Check sheet for the modelled part. Datum: model origin and axes. Units: mm. Face numbers are marked on the shaded views. A direction names the side the tool comes from. Coordinates: 2 decimals unless noted, no trailing zeros. Write each loop counter-clockwise with the first axis right and the second up, starting at its lowest first coordinate (ties: lowest second). Pieces come first, ordered by that corner, then holes. Notation, with made-up numbers: M -18,6.25 L 15,6.25 A19 cw 15,36.25 Z; hole C 31,55.25 d2. An arc over 180 degrees is marked long. Answer as CSV lines item,"result".
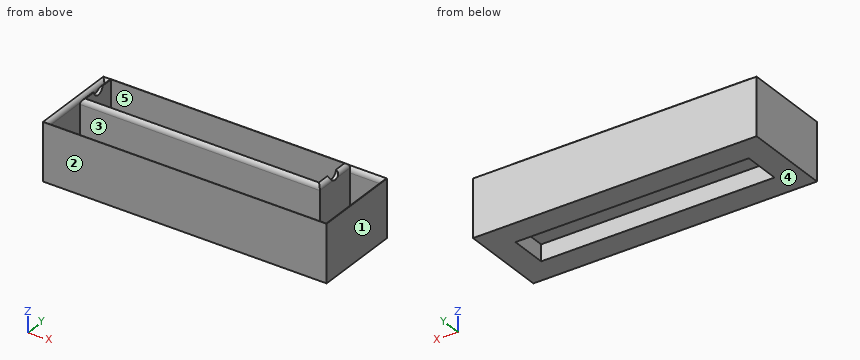
from build123d import *

# Parameters (mm, degrees)
F0_W          = 260
F0_H          = 80
F1_DEPTH      = 1
F2_W          = 10
F2_H          = 10
F3_DEPTH      = 50
F4_T          = 1
F4_T3_DEPTH   = 12
F4_T5_DEPTH   = 12
F4_T7_DEPTH   = 12
F4_T9_DEPTH   = 12
F5_W          = 260
F5_H          = 80
F6_DEPTH      = 3
F7_W          = 260
F7_H          = 80
F7_W_2        = 254
F7_H_2        = 74
F8_DEPTH      = 50
F9_W          = 220
F9_H          = 40
F10_DEPTH     = 67
F11_W         = 214
F11_H         = 34
F12_DEPTH     = 52
F13_W         = 214
F13_H         = 34
F14_DEPTH     = 15
F15_T1_DEPTH  = 245
F15_T3_DEPTH  = 65
F15_T5_DEPTH  = 254
F15_T7_DEPTH  = 74
F15_T13_DEPTH = 86.5
F15_T19_DEPTH = 266.5
F15_T28_DEPTH = 86.5
F15_T34_DEPTH = 266.5
F15_T43_DEPTH = 266.5
F15_T49_DEPTH = 86.5
F15_T58_DEPTH = 86.5
F15_T64_DEPTH = 266.5
F16_R         = 5.7285158572
F17_DEPTH     = 500
F18_W         = 260
F18_H         = 80
F19_DEPTH     = 51


# Not quite as in the source:
# - a fillet or chamfer that OpenCascade refuses, or shapes differently, is made with other operations: its cross-section is extruded or revolved along the edge and cut away or added
# - a shell that OpenCascade refuses in one call is made with other operations: the cavity is built on its own and cut out


with BuildPart() as f1:
    # F0 (on Top) → F1 (new body)
    with BuildSketch(Plane.XY):
        Rectangle(F0_W, F0_H)
    extrude(amount=F1_DEPTH)

    # F2 (on face) → F3 (join)
    with BuildSketch(Plane.XY.offset(1)):
        with Locations((-125, 35)):
            Rectangle(F2_W, F2_H)
        with Locations((125, 35)):
            Rectangle(F2_W, F2_H)
        with Locations((-125, -35)):
            Rectangle(F2_W, F2_H)
        with Locations((125, -35)):
            Rectangle(F2_W, F2_H)
    extrude(amount=F3_DEPTH)

    # F4: shell of thickness 1, made by hand


with BuildPart() as f4_core1:
    # F4_t2: copy of F1
    add(f1.part)

    # the walls: a layer under each face that stays
    f4_faces = [f4_core1.faces().sort_by_distance(p)[0] for p in [
        (121.3333333333, 40, 49.3),
        (-121.3333333333, -40, 49.3),
        (125, -35, 51),
        (125, -30, 26),
        (120, -35, 26),
        (-120, -35, 26),
        (-125, -30, 26),
        (-125, -35, 51),
        (-130, 34.2857142857, 47.3571428571),
        (-125, 30, 26),
        (-125, 35, 51),
        (-120, 35, 26),
        (0, 0, 1),
        (125, 30, 26),
        (120, 35, 26),
        (125, 35, 51),
        (130, -34.2857142857, 47.3571428571),
    ]]
    thicken(f4_faces, amount=-F4_T, mode=Mode.SUBTRACT)

    # F4_s4 → F4_t3 (cut)
    with BuildSketch(Plane.YZ.offset(119)):
        Polygon((-29.99, 1.01), (-31, 1), (-31, 0), (-30, 0), align=None)
        Polygon((29.99, 1.01), (30, 0), (31, 0), (31, 1), align=None)
    extrude(amount=F4_T3_DEPTH, mode=Mode.SUBTRACT)

    # F4_s6 → F4_t5 (cut)
    with BuildSketch(Plane.XZ.offset(29)):
        Polygon((119.99, 1.01), (121, 1), (121, 0), (120, 0), align=None)
        Polygon((-119.99, 1.01), (-121, 1), (-121, 0), (-120, 0), align=None)
    extrude(amount=F4_T5_DEPTH, mode=Mode.SUBTRACT)

    # F4_s8 → F4_t7 (cut)
    with BuildSketch(Plane.YZ.offset(-131)):
        Polygon((-29.99, 1.01), (-31, 1), (-31, 0), (-30, 0), align=None)
        Polygon((29.99, 1.01), (31, 1), (31, 0), (30, 0), align=None)
    extrude(amount=F4_T7_DEPTH, mode=Mode.SUBTRACT)

    # F4_s10 → F4_t9 (cut)
    with BuildSketch(Plane.XZ.offset(-41)):
        Polygon((-119.99, 1.01), (-121, 1), (-121, 0), (-120, 0), align=None)
        Polygon((119.99, 1.01), (120, 0), (121, 0), (121, 1), align=None)
    extrude(amount=F4_T9_DEPTH, mode=Mode.SUBTRACT)


with BuildPart() as f1_1:
    add(f1.part)

    # what is left inside the walls is the cavity
    f4_cavity = [f4_core1.part.solids().sort_by_distance(p)[0] for p in [
        (125, 38.99, 33.333333),
        (-125, 38.99, 33.333333),
        (128.99, -35, 33.333333),
        (-123.666667, -31.01, 25),
    ]]
    add(f4_cavity, mode=Mode.SUBTRACT)

    # F5 (on face) → F6 (join)
    with BuildSketch(Plane.XY.offset(51)):
        Rectangle(F5_W, F5_H)
    extrude(amount=F6_DEPTH)

    # F7 (on face) → F8 (join)
    with BuildSketch(Plane.XY.offset(54)):
        Rectangle(F7_W, F7_H)
        Rectangle(F7_W_2, F7_H_2, mode=Mode.SUBTRACT)
    extrude(amount=F8_DEPTH)

    # F9 (on face) → F10 (join)
    with BuildSketch(Plane.XY.offset(54)):
        Rectangle(F9_W, F9_H)
    extrude(amount=F10_DEPTH)

    # F11 (on face) → F12 (cut)
    with BuildSketch(Plane.XY.offset(121)):
        Rectangle(F11_W, F11_H)
    extrude(amount=-F12_DEPTH, mode=Mode.SUBTRACT)

    # F13 (on face) → F14 (cut)
    with BuildSketch(Plane(origin=(0, 0, 51), x_dir=(1, 0, 0), z_dir=(0, 0, -1))):
        Rectangle(F13_W, F13_H)
    extrude(amount=-F14_DEPTH, mode=Mode.SUBTRACT)

    # F15: fillet of radius 5 on 8 edges, made by hand

    # F15_s2 → F15_t1 (cut)
    with BuildSketch(Plane.YZ.offset(-122.5)):
        with BuildLine():
            ThreePointArc((-20, 116), (-18.5355339059, 119.5355339059), (-15, 121))
            Line((-15, 121), (-20, 121))
            Line((-20, 121), (-20, 116))
        make_face()
        with BuildLine():
            ThreePointArc((20, 116), (18.5355339059, 119.5355339059), (15, 121))
            Line((15, 121), (20, 121))
            Line((20, 121), (20, 116))
        make_face()
    extrude(amount=F15_T1_DEPTH, mode=Mode.SUBTRACT)

    # F15_s4 → F15_t3 (cut)
    with BuildSketch(Plane.XZ.offset(-32.5)):
        with BuildLine():
            ThreePointArc((-110, 116), (-108.5355339059, 119.5355339059), (-105, 121))
            Line((-105, 121), (-110, 121))
            Line((-110, 121), (-110, 116))
        make_face()
        with BuildLine():
            ThreePointArc((110, 116), (108.5355339059, 119.5355339059), (105, 121))
            Line((105, 121), (110, 121))
            Line((110, 121), (110, 116))
        make_face()
    extrude(amount=F15_T3_DEPTH, mode=Mode.SUBTRACT)

    # F15_s6 → F15_t5 (cut)
    with BuildSketch(Plane.YZ.offset(-127)):
        with BuildLine():
            ThreePointArc((-42, 104), (-38.4644660941, 102.5355339059), (-37, 99))
            Line((-37, 99), (-37, 104))
            Line((-37, 104), (-42, 104))
        make_face()
        with BuildLine():
            ThreePointArc((42, 104), (38.4644660941, 102.5355339059), (37, 99))
            Line((37, 99), (37, 104))
            Line((37, 104), (42, 104))
        make_face()
    extrude(amount=F15_T5_DEPTH, mode=Mode.SUBTRACT)

    # F15_s8 → F15_t7 (cut)
    with BuildSketch(Plane.XZ.offset(-37)):
        with BuildLine():
            ThreePointArc((132, 104), (128.4644660941, 102.5355339059), (127, 99))
            Line((127, 99), (127, 104))
            Line((127, 104), (132, 104))
        make_face()
        with BuildLine():
            ThreePointArc((-132, 104), (-128.4644660941, 102.5355339059), (-127, 99))
            Line((-127, 99), (-127, 104))
            Line((-127, 104), (-132, 104))
        make_face()
    extrude(amount=F15_T7_DEPTH, mode=Mode.SUBTRACT)


with BuildPart() as f15_tool11:
    # F15_s12 → F15_t13 (new body)
    with BuildSketch(Plane.XZ.offset(-37)):
        with BuildLine():
            ThreePointArc((132, 104), (128.4644660941, 102.5355339059), (127, 99))
            Line((127, 99), (127, 104))
            Line((127, 104), (132, 104))
        make_face()
    extrude(amount=F15_T13_DEPTH)

    split(bisect_by=Plane.YZ.offset(130), keep=Keep.BOTTOM)

    split(bisect_by=Plane.XZ.offset(40), keep=Keep.BOTTOM)

    split(bisect_by=Plane.XZ.offset(37), keep=Keep.TOP)


with BuildPart() as f15_tool17:
    # F15_s18 → F15_t19 (new body)
    with BuildSketch(Plane.YZ.offset(139.5)):
        with BuildLine():
            ThreePointArc((-42, 104), (-38.4644660941, 102.5355339059), (-37, 99))
            Line((-37, 99), (-37, 104))
            Line((-37, 104), (-42, 104))
        make_face()
    extrude(amount=-F15_T19_DEPTH)

    split(bisect_by=Plane.YZ.offset(130), keep=Keep.BOTTOM)

    split(bisect_by=Plane.XZ.offset(40), keep=Keep.BOTTOM)

    split(bisect_by=Plane.YZ.offset(127), keep=Keep.TOP)


with BuildPart() as f15_tool11_1:
    add(f15_tool11.part)

    # F15_t23: intersect F15_tool17
    add(f15_tool17.part, mode=Mode.INTERSECT)


with BuildPart() as f1_2:
    add(f1_1.part)

    # F15_t9: cut F15_tool11
    add(f15_tool11_1.part, mode=Mode.SUBTRACT)


with BuildPart() as f15_tool26:
    # F15_s27 → F15_t28 (new body)
    with BuildSketch(Plane.XZ.offset(49.5)):
        with BuildLine():
            ThreePointArc((-132, 104), (-128.4644660941, 102.5355339059), (-127, 99))
            Line((-127, 99), (-127, 104))
            Line((-127, 104), (-132, 104))
        make_face()
    extrude(amount=-F15_T28_DEPTH)

    split(bisect_by=Plane.YZ.offset(-130), keep=Keep.TOP)

    split(bisect_by=Plane.XZ.offset(40), keep=Keep.BOTTOM)

    split(bisect_by=Plane.XZ.offset(37), keep=Keep.TOP)


with BuildPart() as f15_tool32:
    # F15_s33 → F15_t34 (new body)
    with BuildSketch(Plane.YZ.offset(127)):
        with BuildLine():
            ThreePointArc((-42, 104), (-38.4644660941, 102.5355339059), (-37, 99))
            Line((-37, 99), (-37, 104))
            Line((-37, 104), (-42, 104))
        make_face()
    extrude(amount=-F15_T34_DEPTH)

    split(bisect_by=Plane.YZ.offset(-130), keep=Keep.TOP)

    split(bisect_by=Plane.XZ.offset(40), keep=Keep.BOTTOM)

    split(bisect_by=Plane.YZ.offset(-127), keep=Keep.BOTTOM)


with BuildPart() as f15_tool26_1:
    add(f15_tool26.part)

    # F15_t38: intersect F15_tool32
    add(f15_tool32.part, mode=Mode.INTERSECT)


with BuildPart() as f1_3:
    add(f1_2.part)

    # F15_t24: cut F15_tool26
    add(f15_tool26_1.part, mode=Mode.SUBTRACT)


with BuildPart() as f15_tool41:
    # F15_s42 → F15_t43 (new body)
    with BuildSketch(Plane.YZ.offset(-127)):
        with BuildLine():
            ThreePointArc((42, 104), (38.4644660941, 102.5355339059), (37, 99))
            Line((37, 99), (37, 104))
            Line((37, 104), (42, 104))
        make_face()
    extrude(amount=F15_T43_DEPTH)

    split(bisect_by=Plane.XZ.offset(-40), keep=Keep.TOP)

    split(bisect_by=Plane.YZ.offset(130), keep=Keep.BOTTOM)

    split(bisect_by=Plane.YZ.offset(127), keep=Keep.TOP)


with BuildPart() as f15_tool47:
    # F15_s48 → F15_t49 (new body)
    with BuildSketch(Plane.XZ.offset(-49.5)):
        with BuildLine():
            ThreePointArc((132, 104), (128.4644660941, 102.5355339059), (127, 99))
            Line((127, 99), (127, 104))
            Line((127, 104), (132, 104))
        make_face()
    extrude(amount=F15_T49_DEPTH)

    split(bisect_by=Plane.XZ.offset(-40), keep=Keep.TOP)

    split(bisect_by=Plane.YZ.offset(130), keep=Keep.BOTTOM)

    split(bisect_by=Plane.XZ.offset(-37), keep=Keep.BOTTOM)


with BuildPart() as f15_tool41_1:
    add(f15_tool41.part)

    # F15_t53: intersect F15_tool47
    add(f15_tool47.part, mode=Mode.INTERSECT)


with BuildPart() as f1_4:
    add(f1_3.part)

    # F15_t39: cut F15_tool41
    add(f15_tool41_1.part, mode=Mode.SUBTRACT)


with BuildPart() as f15_tool56:
    # F15_s57 → F15_t58 (new body)
    with BuildSketch(Plane.XZ.offset(37)):
        with BuildLine():
            ThreePointArc((-132, 104), (-128.4644660941, 102.5355339059), (-127, 99))
            Line((-127, 99), (-127, 104))
            Line((-127, 104), (-132, 104))
        make_face()
    extrude(amount=-F15_T58_DEPTH)

    split(bisect_by=Plane.XZ.offset(-40), keep=Keep.TOP)

    split(bisect_by=Plane.YZ.offset(-130), keep=Keep.TOP)

    split(bisect_by=Plane.XZ.offset(-37), keep=Keep.BOTTOM)


with BuildPart() as f15_tool62:
    # F15_s63 → F15_t64 (new body)
    with BuildSketch(Plane.YZ.offset(-139.5)):
        with BuildLine():
            ThreePointArc((42, 104), (38.4644660941, 102.5355339059), (37, 99))
            Line((37, 99), (37, 104))
            Line((37, 104), (42, 104))
        make_face()
    extrude(amount=F15_T64_DEPTH)

    split(bisect_by=Plane.XZ.offset(-40), keep=Keep.TOP)

    split(bisect_by=Plane.YZ.offset(-130), keep=Keep.TOP)

    split(bisect_by=Plane.YZ.offset(-127), keep=Keep.BOTTOM)


with BuildPart() as f15_tool56_1:
    add(f15_tool56.part)

    # F15_t68: intersect F15_tool62
    add(f15_tool62.part, mode=Mode.INTERSECT)


with BuildPart() as f1_5:
    add(f1_4.part)

    # F15_t54: cut F15_tool56
    add(f15_tool56_1.part, mode=Mode.SUBTRACT)

    # F16 (on face) → F17 (cut)
    with BuildSketch(Plane.YZ.offset(110)):
        with Locations((0, 121.0692673922)):
            Circle(F16_R)
    extrude(amount=-F17_DEPTH, mode=Mode.SUBTRACT)

    # F18 (on face) → F19 (cut)
    with BuildSketch(Plane(origin=(0, 0, 0), x_dir=(1, 0, 0), z_dir=(0, 0, -1))):
        Rectangle(F18_W, F18_H)
    extrude(amount=-F19_DEPTH, mode=Mode.SUBTRACT)


solid = f1_5.part
1) Tool access check on the marked faces 4 and 5. Record the directions out of +Z, -Z, +X, -X, +Y, -Y that give a thin tool (end or side, any length) a straight path to the whole face; none if there is none.
Answer key:
face 4,"-Z, +X, -X, +Y, -Y"
face 5,"+Z"
2) Section check A-A, the plane z = 79.5. Record the boundary of the cut face in (x, y), plus the area to 3 significant figures.
Answer key:
outline,"M -130,-40 L 130,-40 L 130,40 L -130,40 Z; M -110,-20 L 110,-20 L 110,20 L -110,20 Z; hole M -127,-37 L 127,-37 L 127,37 L -127,37 Z; hole M -107,-17 L 107,-17 L 107,17 L -107,17 Z"
area,"3,530 mm2"
3) Thickness scan on line 1 along Y through (x, z) = (-68, 58); line 2 along X through (y, z) = (-5, 80.5); line 3 along X through (y, z) = (7, 112.5). Record the ranges inside material, lowest first.
Answer key:
line 1,"y = -40 to -37, -20 to -17, 17 to 20, 37 to 40"
line 2,"x = -130 to -127, -110 to -107, 107 to 110, 127 to 130"
line 3,"x = -110 to -107, 107 to 110"
4) Mould release check, pull along Y, two halves, no side actions. Record for the marked faces 1, 2 and 3: pulls with the +Y half, pulls with the -Y half, needs draft (parallel to the pull), parting line crosses it, or undercut.
Answer key:
face 1,"needs draft"
face 2,"pulls with the -Y half"
face 3,"undercut"
5) Section check C-C, the plane x = -112.5. Record the boundary of the cut face in (y, z).
Answer key:
outline,"M -40,51 L 40,51 L 40,103.58 A5 ccw 37,99 L 37,54 L -37,54 L -37,99 A5 ccw -40,103.58 Z"
6) Section check B-B, the plane y = -28. Record the boundary of the cut face in (x, z).
Answer key:
outline,"M -130,51 L 130,51 L 130,103.58 A5 ccw 127,99 L 127,54 L -127,54 L -127,99 A5 ccw -130,103.58 Z"
7) Depth check by flat-ended pin: P1, Ø4, axis at x = 15.5, z = 112.5, coming from the +Y side; P2, Ø8, axis at x = -13.5, y = 4, coming from the -Z side; P3, Ø8, axis at y = -6, z = 112, coming from the -X side. Enter the tip coordinate at first touch or a pass-through.
Answer key:
P1,"stops at y = 20"
P2,"stops at z = 66"
P3,"stops at x = -110"
8) Section check D-D, the plane y = 10. Record the boundary of the cut face in (x, z), plus the area to 3 significant figures.
Answer key:
outline,"M -130,51 L -107,51 L -107,66 L 107,66 L 107,51 L 130,51 L 130,103.58 A5 ccw 127,99 L 127,54 L 110,54 L 110,116 A5 ccw 107,120.58 L 107,69 L -107,69 L -107,120.58 A5 ccw -110,116 L -110,54 L -127,54 L -127,99 A5 ccw -130,103.58 Z"
area,"1,460 mm2"
